Source: three-view drawing plus pictorial views. Frame: mm from the lowest corner of the part. Give positions to 0.01 mm unless a question says otherwise; leave off trailing zeros. Loops run counter-clockwise (first coordinate to the right, second up) from the corner with the lowest first, then second, coordinate; pieces in that order, holes last. Notation, with made-up numbers: (-14.75, 14) - (32.25, 14) arc R27 cw to (32.25, 36) - close; hole circle Ø10 at (78.25, 60). An arc over 180 degrees is marked (long way). One line per item, written item: value.
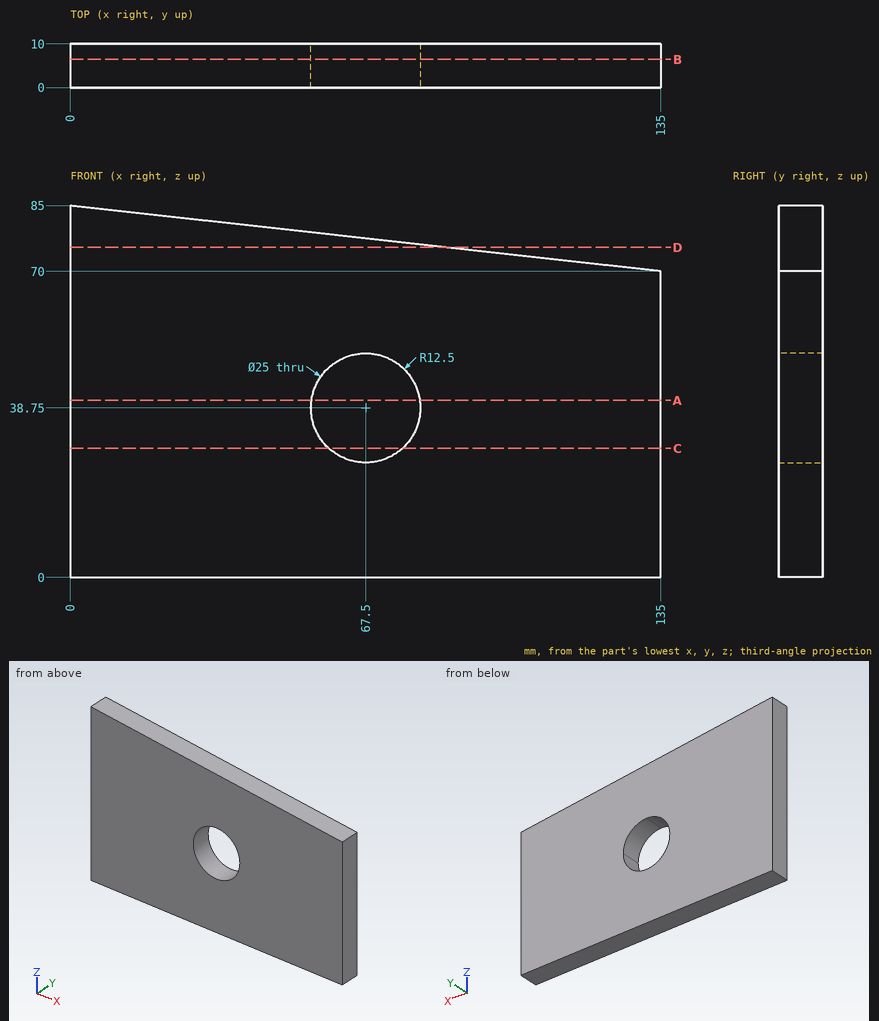
Item 1: Section B-B, the plane y = 6.5. Output: boundary loops of the cut face in (x, z), and give its area (3 significant figures).
Verdict:
outline: (0, 0) - (135, 0) - (135, 70) - (0, 85) - close; hole circle Ø25 at (67.5, 38.75)
area: 9,970 mm^2
Item 2: Section D-D, the plane z = 75.5. Output: boundary loops of the cut face in (x, y).
Verdict:
outline: (0, 0) - (85.5, 0) - (85.5, 10) - (0, 10) - close
Item 3: Material intervals for L1, parallel to X at y = 5.5, z = 38.5; L2, parallel to X at y = 4.5, z = 47; L3, parallel to Z at x = 67.5, y = 4, sorted ascending.
Verdict:
L1: x = 0 to 55, 80 to 135
L2: x = 0 to 58.11, 76.89 to 135
L3: z = 0 to 26.25, 51.25 to 77.5
Item 4: Pin query (flat end, axial travel): P1, Ø4, axis at x = 17, y = 2.5, coming from the +Z side. Return the tip coordinate at first contact, or that it passes through.
Verdict:
P1: stops at z = 83.33
Item 5: Section C-C, the plane z = 29.5. Output: boundary loops of the cut face in (x, y), and give its area (3 significant figures).
Verdict:
outline: (0, 0) - (59.09, 0) - (59.09, 10) - (0, 10) - close; (75.91, 0) - (135, 0) - (135, 10) - (75.91, 10) - close
area: 1,180 mm^2
Item 6: Section A-A, the plane z = 40.5. Output: boundary loops of the cut face in (x, y).
Verdict:
outline: (0, 0) - (55.12, 0) - (55.12, 10) - (0, 10) - close; (79.88, 0) - (135, 0) - (135, 10) - (79.88, 10) - close
